Geometry: final body of the model. Coordinates: model frame, mm. A direction names the side the tool comes from. Coordinates: 2 decimals unless noted, no trailing zeros. Order: outer loops, then holes, each group sorted by start corner. A loop starts at its lowest first (then second) coordinate and runs counter-clockwise, first axis right, second up. Notation, with made-up numbers: (57.5, -6.75) - (114.5, -6.75) arc R13 cw to (114.5, -0.75) - close; hole circle Ø11 at (3, -8). An arc over 180 degrees is marked (long way). Use a Markdown table: item, result. Add a question column.
```python
from build123d import *

# Parameters (mm, degrees)
RESSALTO_EXTRUS_O1_DEPTH = 2
ESBO_O2_R                = 1.65
ESBO_O2_R_2              = 1.5
ESBO_O2_R_3              = 1
CORTE_EXTRUS_O1_DEPTH    = 3.0000001


with BuildPart() as part:
    # Esboço1 → Ressalto-extrusão1 (new body)
    with BuildSketch(Plane(origin=(0, 0, 0), x_dir=(1, 0, 0), z_dir=(0, 1, 0))):
        with BuildLine():
            Line((-57, 14.836150135), (-51, 9.5))
            Line((-51, 9.5), (-22.083647797, 9.5))
            add(Edge.make_bspline(
                [(22.083647797, 9.5), (0, 38), (-22.083647797, 9.5)],
                knots=[0.523598776, 0.523598776, 0.523598776, 2.617993878, 2.617993878, 2.617993878], degree=2, weights=[1, 0.5, 1]))
            Line((22.083647797, 9.5), (51, 9.5))
            Line((51, 9.5), (57, 14.836150135))
            Line((57, 14.836150135), (68, 14.836150135))
            Line((68, 14.836150135), (68, 8.836150135))
            Line((68, 8.836150135), (70, 8.836150135))
            Line((70, 8.836150135), (70, -7.163849865))
            Line((70, -7.163849865), (68, -7.163849865))
            Line((68, -7.163849865), (68, -13.163849865))
            Line((68, -13.163849865), (57, -13.163849865))
            Line((57, -13.163849865), (51, -9.5))
            Line((51, -9.5), (22.083647797, -9.5))
            add(Edge.make_bspline(
                [(-22.083647797, -9.5), (0, -38), (22.083647797, -9.5)],
                knots=[3.665191429, 3.665191429, 3.665191429, 5.759586532, 5.759586532, 5.759586532], degree=2, weights=[1, 0.5, 1]))
            Line((-22.083647797, -9.5), (-51, -9.5))
            Line((-51, -9.5), (-57, -13.163849865))
            Line((-57, -13.163849865), (-68, -13.163849865))
            Line((-68, -13.163849865), (-68, -7.163849865))
            Line((-68, -7.163849865), (-70, -7.163849865))
            Line((-70, -7.163849865), (-70, 8.836150135))
            Line((-70, 8.836150135), (-68, 8.836150135))
            Line((-68, 8.836150135), (-68, 14.836150135))
            Line((-68, 14.836150135), (-57, 14.836150135))
        make_face()
    extrude(amount=RESSALTO_EXTRUS_O1_DEPTH)

    # Esboço2 → Corte-extrusão1 (cut, through all)
    with BuildSketch(Plane(origin=(0, 2, 0), x_dir=(1, 0, 0), z_dir=(0, 1, 0))):
        with Locations((0, 15)):
            Circle(ESBO_O2_R)
        with Locations((10, 10.4)):
            Circle(ESBO_O2_R_2)
        with Locations((-10, 10.4)):
            Circle(ESBO_O2_R_2)
        with Locations((0, -15)):
            Circle(ESBO_O2_R)
        with Locations((10, -10.4)):
            Circle(ESBO_O2_R_2)
        with Locations((-10, -10.4)):
            Circle(ESBO_O2_R_2)
        with Locations((-10, 0)):
            Circle(ESBO_O2_R_3)
        with Locations((18, 0)):
            Circle(ESBO_O2_R_3)
        with BuildLine():
            Line((25, 3.836150135), (61, 3.836150135))
            ThreePointArc((61, 3.836150135), (61.707106781, 3.543256916), (62, 2.836150135))
            Line((62, 2.836150135), (62, -1.163849865))
            ThreePointArc((62, -1.163849865), (61.707106781, -1.870956646), (61, -2.163849865))
            Line((61, -2.163849865), (25, -2.163849865))
            ThreePointArc((25, -2.163849865), (24.292893219, -1.870956646), (24, -1.163849865))
            Line((24, -1.163849865), (24, 2.836150135))
            ThreePointArc((24, 2.836150135), (24.292893219, 3.543256916), (25, 3.836150135))
        make_face()
        with BuildLine():
            Line((-61, 3.836150135), (-25, 3.836150135))
            ThreePointArc((-25, 3.836150135), (-24.292893219, 3.543256916), (-24, 2.836150135))
            Line((-24, 2.836150135), (-24, -1.163849865))
            ThreePointArc((-24, -1.163849865), (-24.292893219, -1.870956646), (-25, -2.163849865))
            Line((-25, -2.163849865), (-61, -2.163849865))
            ThreePointArc((-61, -2.163849865), (-61.707106781, -1.870956646), (-62, -1.163849865))
            Line((-62, -1.163849865), (-62, 2.836150135))
            ThreePointArc((-62, 2.836150135), (-61.707106781, 3.543256916), (-61, 3.836150135))
        make_face()
        with BuildLine():
            Line((-7, 7), (15, 7))
            ThreePointArc((15, 7), (15.707106781, 6.707106781), (16, 6))
            Line((16, 6), (16, -6))
            ThreePointArc((16, -6), (15.707106781, -6.707106781), (15, -7))
            Line((15, -7), (-7, -7))
            ThreePointArc((-7, -7), (-7.707106781, -6.707106781), (-8, -6))
            Line((-8, -6), (-8, 6))
            ThreePointArc((-8, 6), (-7.707106781, 6.707106781), (-7, 7))
        make_face()
    extrude(amount=-CORTE_EXTRUS_O1_DEPTH, mode=Mode.SUBTRACT)


solid = part.part
```
1) Section B-B (y = 0.35). Give the number of separate pieces and of enclosed holes in the cut face, then the cut area to 3 significant figures.
2) Set-up query: faces 1 (the face through (-53.958, 0.986, 11.306)), 2 (the face through (8.89, 1.01, -11.41)), 3 (the face through (-54.042, 0.986, -12.205)). Return all of +Z, -Z, +X, -X, +Y, -Y with unobstructed straight access to the full face (end or side cutting, diameter ignored); none if empty.
3) Pin query (flat end, axial travel): pin 1 (2.5 mm diameter, centred on x = -10, z = 10.4, fed in from +Y); pin 2 (1 mm diameter, centred on x = -69.5, y = 0.5, fed in from -Z); pin 3 (1 mm diameter, centred on y = 1, z = 11.5, fed in from -X); pin 4 (1 mm diameter, centred on x = 36.5, y = 1, fed in from +Z). Return the tip coordinate at first contact, or that it passes through.
4) Ray query, line 1 along Z through (x, y) = (0, 0.7); line 2 along Z through (x, y) = (-43.5, 0.7); line 3 along X through (y, z) = (1.5, -3). Return the intervals inside material, ascending.
5) Draft query along Z for faces 4 (the face through (54.042, 0.986, 11.358)), 5 (the face through (53.96, 0.99, -12.13)), 6 (the face through (8.89, 1.01, 9.39)). Return one class per face: pulls with the +Z half, pulls with the -Z half, needs draft (parallel to the pull), parting line crosses it, or undercut.
6) Section A-A (x = -32). Return loops of the section in (y, z).
Values follow:
| question | item | result |
|---|---|---|
| 1 | separate pieces | 1 |
| 1 | enclosed holes | 11 |
| 1 | area | 2,650 mm² |
| 2 | face 1 | +Z, +Y, -Y |
| 2 | face 2 | +Y, -Y |
| 2 | face 3 | -Z, +Y, -Y |
| 3 | pin 1 | passes through |
| 3 | pin 2 | stops at z = -8.84 |
| 3 | pin 3 | stops at x = -68 |
| 3 | pin 4 | stops at z = 9.5 |
| 4 | line 1 | z = -19 to -16.65, -13.35 to -7, 7 to 13.35, 16.65 to 19 |
| 4 | line 2 | z = -9.5 to -3.84, 2.16 to 9.5 |
| 4 | line 3 | x = -70 to -61.99, -24.01 to -8, 16 to 24.01, 61.99 to 70 |
| 5 | face 4 | pulls with the +Z half |
| 5 | face 5 | pulls with the -Z half |
| 5 | face 6 | undercut |
| 6 | outline | (0, -9.5) - (2, -9.5) - (2, -3.84) - (0, -3.84) - close; (0, 2.16) - (2, 2.16) - (2, 9.5) - (0, 9.5) - close |
